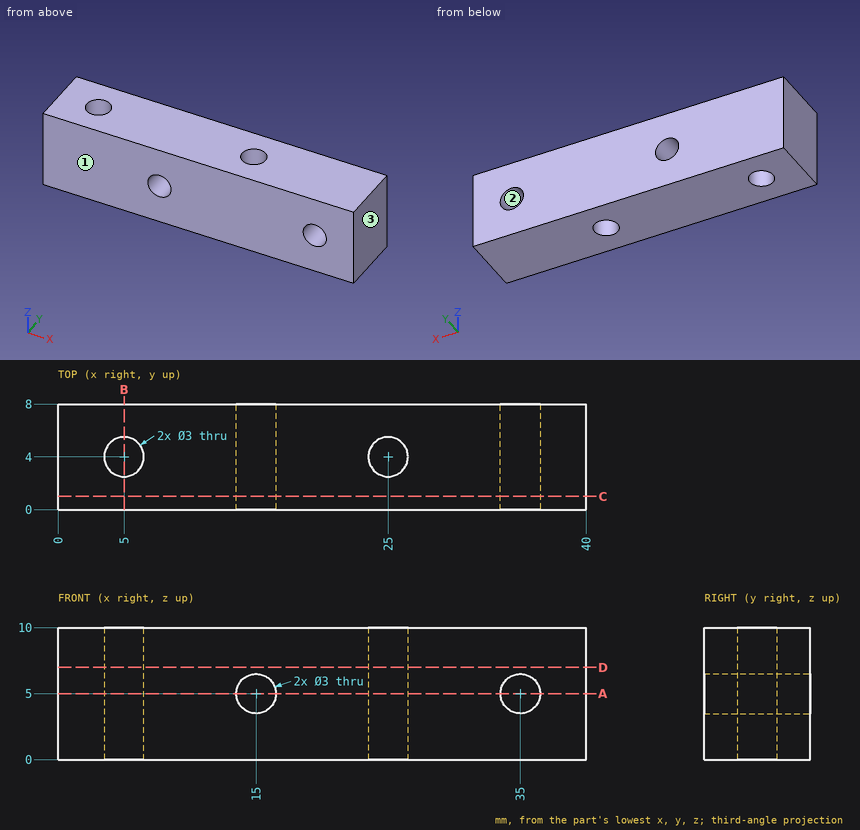
Print and shaded views of the part. All mm, measured from the part's lowest x, y and z. Round coordinates to 2 decimals unless told otherwise and drop trailing zeros. Order: outer loops, then holes, each group sorted by start corner. A loop starts at its lowest first (then second) coordinate and runs counter-clockwise, first axis right, second up.
Q1. Slice it at B-B (x = 5). Write the cut outline in (y, z), and give its area (3 significant figures).
Q2. Wall check: L1, parallel to X at y = 2, z = 5; L2, parallel to Z at x = 15, y = 3; L3, parallel to X at y = 4.5, z = 7.75. Give the ranges that are in metal, low to high.
Q3. Slice it at A-A (z = 5). Write the cut outline in (x, y).
Q4. Slice it at D-D (z = 7). Write the cut outline in (x, y).
Q5. Two-plate mould, pull along X, no slides. Class the marked faces 1, 2 and 3: pulls with the +X half, pulls with the -X half, needs draft (parallel to the pull), parting line crosses it, or undercut.
Q6. Slice it at C-C (y = 1). Write the cut outline in (x, z), and give its area (3 significant figures).
Q7. Drop flat-ended pins along their axis: pin 1 (2.5 mm diameter, centred on x = 15, z = 5, fed in from -Y); pin 2 (4 mm diameter, centred on y = 1, z = 8.5, fed in from -X). Give the stop position or say it passes through.
Results below:
1. outline: (0, 0) - (2.5, 0) - (2.5, 10) - (0, 10) - close; (5.5, 0) - (8, 0) - (8, 10) - (5.5, 10) - close
1. area: 50.0 mm2
2. L1: x = 0 to 13.5, 16.5 to 33.5, 36.5 to 40
2. L2: z = 0 to 3.5, 6.5 to 10
2. L3: x = 0 to 3.59, 6.41 to 23.59, 26.41 to 40
3. outline: (0, 0) - (13.5, 0) - (13.5, 8) - (0, 8) - close; (16.5, 0) - (33.5, 0) - (33.5, 8) - (16.5, 8) - close; (36.5, 0) - (40, 0) - (40, 8) - (36.5, 8) - close; hole circle Ø3 at (5, 4); hole circle Ø3 at (25, 4)
4. outline: (0, 0) - (40, 0) - (40, 8) - (0, 8) - close; hole circle Ø3 at (5, 4); hole circle Ø3 at (25, 4)
5. face 1: needs draft
5. face 2: undercut
5. face 3: pulls with the +X half
6. outline: (0, 0) - (40, 0) - (40, 10) - (0, 10) - close; hole circle Ø3 at (15, 5); hole circle Ø3 at (35, 5)
6. area: 386 mm2
7. pin 1: passes through
7. pin 2: stops at x = 0
